from build123d import *

# Parameters (mm, degrees)
CUT_EXTRUDE1_DEPTH = 2.54
M2_TAPPED_HOLE1_D  = 1.6


with BuildPart() as part:
    # Sketch1 → Revolve1 (revolve)
    with BuildSketch(Plane.XY, mode=Mode.PRIVATE) as revolve1_sk:
        with BuildLine():
            Line((0, 0), (0, 5.7))
            Line((0, 5.7), (-1.5, 5.7))
            ThreePointArc((-1.5, 5.7), (-2.5, 3.7), (-1.5, 1.7))
            Line((-1.5, 1.7), (-1.5, 0.95))
            Line((-1.5, 0.95), (-2.25, 0.5))
            Line((-2.25, 0.5), (-2.25, 0))
            Line((-2.25, 0), (0, 0))
        make_face()
    revolve(revolve1_sk.sketch.rotate(Axis((0, 0, 0), (0, 1, 0)), 270), axis=Axis((0, 0, 0), (0, 1, 0)))

    # Sketch2 → Cut-Extrude1 (cut)
    with BuildSketch(Plane(origin=(0, 5.7, 0), x_dir=(1, 0, 0), z_dir=(0, 1, 0))):
        Polygon((-1, -0.577350269), (-1, 0.577350269), (0, 1.154700538), (1, 0.577350269), (1, -0.577350269), (0, -1.154700538), align=None)
    extrude(amount=-CUT_EXTRUDE1_DEPTH, mode=Mode.SUBTRACT)

    # M2 Tapped Hole1 (through all)
    with Locations(Plane(origin=(0, 0, 0), x_dir=(-1, 0, 0), z_dir=(0, -1, 0))):
        with Locations((0, 0)):
            Hole(M2_TAPPED_HOLE1_D / 2)


solid = part.part
Check sheet for the modelled part. Datum: model origin and axes. Units: mm. A direction names the side the tool comes from. Give positions to 0.01 mm unless a question says otherwise; leave off trailing zeros. Loops run counter-clockwise (first coordinate to the right, second up) from the corner with the lowest first, then second, coordinate; pieces in that order, holes last. Notation, with made-up numbers: M 83.5,-34 L 94.5,-34 A18 cw 94.5,-22 Z; hole C -22.75,30 d6. An arc over 180 degrees is marked long. Return JSON: item names as keys, results as strings. Group by question number.
1. Go/stop test with flat-tipped pins: pin 1 (0.6 mm diameter, centred on y = 4.5, z = 0, fed in from -X); pin 2 (2 mm diameter, centred on y = 3, z = 1, fed in from -X). Record where each tip stops, or that it passes through.
2. Tool access check on faces 4 (the cylindrical face through (-0.63, 1.6, 0.49)), 5 (the cylindrical face through (-0.676, 0.246, -2.146)), 6 (the flat face through (-0.49, 4.45, 0.87)). Record the directions out of +Z, -Z, +X, -X, +Y, -Y that give a thin tool (end or side, any length) a straight path to the whole face; none if there is none.
3. Cross-section at A-A on z = 0. Record the boundary of the cut face in (x, y).
4. Cross-section at B-B on y = 4.7. Record the boundary of the cut face in (x, z).
5. Mould release check, pull along Y, two halves, no side actions. Record for faces 1 (the flat face through (1, 4, 0)), 2 (the cylindrical face through (-0.45, 1.32, -1.43)), 3 (the flat face through (1, 0, 0)): released by +Y, released by -Y, zero draft, split by the parting line, or undercut.
6. Cross-section at C-C on y = 0.8. Record the boundary of the cut face in (x, z).
7. Cross-section at D-D on y = 3. Record the boundary of the cut face in (x, z), plus the area to 3 significant figures.
8. Thickness scan on L1, parallel to Y at x = 0.6, z = -1.6; L2, parallel to Z at x = -0.3, y = 3.8; L3, parallel to Z at x = 0.55, y = 0.6. Record the ranges inside material, lowest first.
Return value:
{
 "1": {"pin 1": "x = -2.45", "pin 2": "x = -2.49"},
 "2": {"face 4": "+Y, -Y", "face 5": "-Y", "face 6": "+Y"},
 "3": {"outline": "M -2.25,0 L -0.8,0 L -0.8,3.16 L -1,3.16 L -1,5.7 L -1.5,5.7 A2.5 ccw -1.5,1.7 L -1.5,0.95 L -2.25,0.5 Z; M 0.8,0 L 2.25,0 L 2.25,0.5 L 1.5,0.95 L 1.5,1.7 A2.5 ccw 1.5,5.7 L 1,5.7 L 1,3.16 L 0.8,3.16 Z"},
 "4": {"outline": "C 0,0 d4.58; hole M -1,-0.58 L 0,-1.15 L 1,-0.58 L 1,0.58 L 0,1.15 L -1,0.58 Z"},
 "5": {"face 1": "zero draft", "face 2": "undercut", "face 3": "released by -Y"},
 "6": {"outline": "C 0,0 d3.5; hole C 0,0 d1.6"},
 "7": {"outline": "C 0,0 d4.8; hole C 0,0 d1.6", "area": "16.1 mm^2"},
 "8": {"L1": "0 to 0.82, 1.88 to 5.52", "L2": "-2.48 to -0.98, 0.98 to 2.48", "L3": "-2.01 to -0.58, 0.58 to 2.01"}
}
